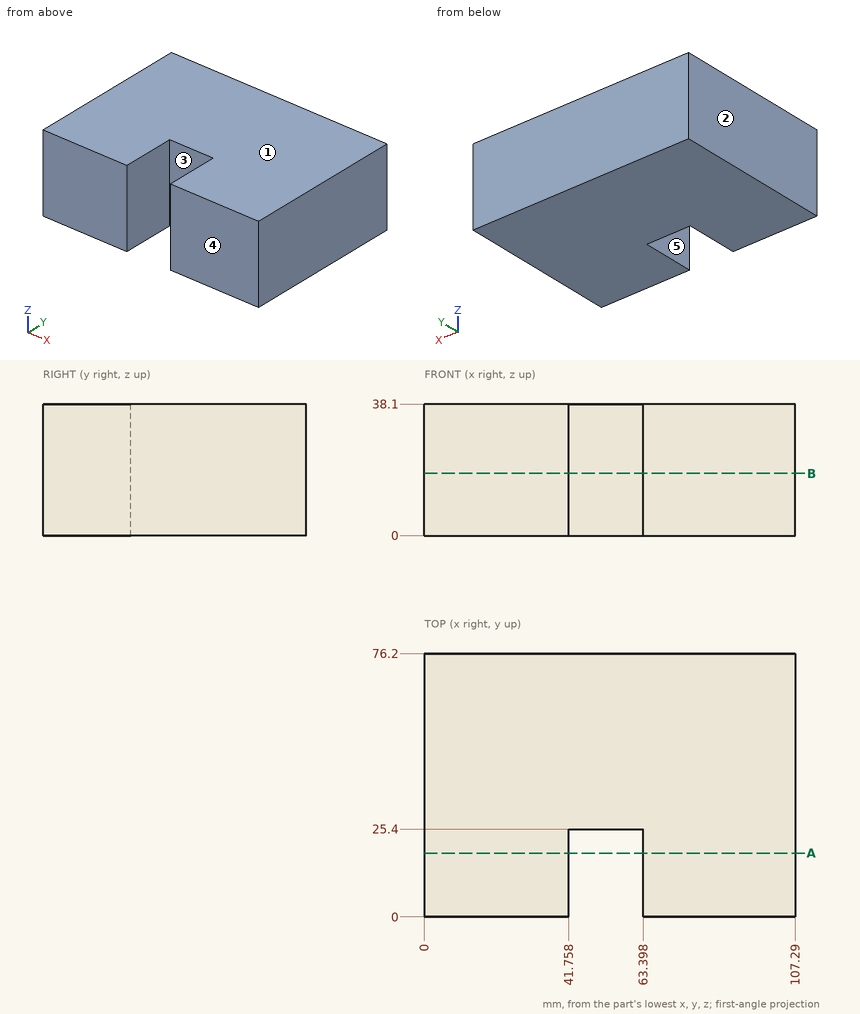
The drawing under review shows one solid part. Ordinate dimensions are in mm from its lowest x, y, z. A direction names the side the tool comes from. Coordinates: 2 decimals unless noted, no trailing zeros. Order: outer loops, then holes, each group sorted by start corner. A loop starts at its lowest first (then second) coordinate and runs counter-clockwise, first axis right, second up. Notation, with made-up numbers: (38.25, -9.75) -> (89.25, -9.75) arc R19 cw to (89.25, -2.75) -> close; hole circle Ø7 at (30.5, 70). An arc over 180 degrees is marked (long way). One line per item, written item: value.
1) We need section A-A, the plane y = 18.5. Give the boundary of the cut face in (x, z), then the cut area to 3 significant figures.
Output values:
outline: (0, 0) -> (41.76, 0) -> (41.76, 38.1) -> (0, 38.1) -> close; (63.4, 0) -> (107.29, 0) -> (107.29, 38.1) -> (63.4, 38.1) -> close
area: 3,260 mm2
2) Machinability: for the marked faces 4 and 5, which of the approach directions +Z, -Z, +X, -X, +Y, -Y give a long, thin tool a straight path to every point of the face, cutting with its end or side? Answer none if there is none.
Output values:
face 4: +Z, -Z, +X, -X, -Y
face 5: +Z, -Z, -Y
3) We need section B-B, the plane z = 18. Give the boundary of the cut face in (x, y).
Output values:
outline: (0, 0) -> (41.76, 0) -> (41.76, 25.4) -> (63.4, 25.4) -> (63.4, 0) -> (107.29, 0) -> (107.29, 76.2) -> (0, 76.2) -> close
4) Draft analysis for pull direction X (two halves, no side actions). For the marked faces 1, 2 and 3, state which applies: +X half, -X half, draft (parallel to the pull), parting line (faces both ways), or undercut.
Output values:
face 1: draft
face 2: -X half
face 3: undercut
5) To check wall thickness, follow probe 1 along X at (y, z) = (11.5, 20); probe 2 along Y at (x, z) = (61.5, 22). State the ranges of each line that lie inside material, in increasing order. Write a range as [from, to].
Output values:
probe 1: x = [0, 41.76], [63.4, 107.29]
probe 2: y = [25.4, 76.2]
6) Clearance check with a flat-ended pin moving along its axis: P1, Ø6.5, axis at x = 53, z = 19.5, coming from the -Y side. State where the tip first meets the part, or that it passes through.
Output values:
P1: stops at y = 25.4
